Read the model definition and answer for the solid it produces. Units are mm, in the model's axes. Face numbers are marked on the shaded views. A direction names the side the tool comes from. Coordinates: 2 decimals unless noted, no trailing zeros. Loops run counter-clockwise (first coordinate to the right, second up) from the corner with the lowest first, then second, coordinate; pieces in that order, holes last.
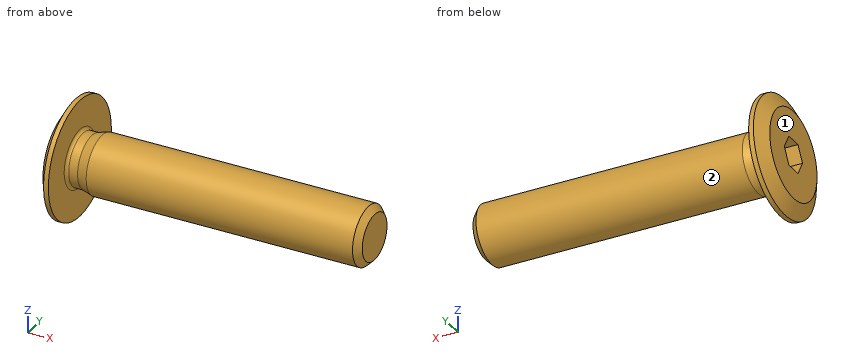
Autodesk Inventor part; units mm, degrees
ref_plane "YZ Plane" through (0, 0, 0) normal (1, 0, 0) x (0, 1, 0)
ref_plane "XZ Plane" through (0, 0, 0) normal (0, 1, 0) x (-1, 0, 0)
ref_plane "XY Plane" through (0, 0, 0) normal (0, 0, 1) x (1, 0, 0)
sketch "Sketch_1" plane through (0, 0, 0) normal (0, 0, 1) x (1, 0, 0)
  line L0 (20, 0) -> (-0.9, 0)
  line L1 (-0.9, 0) -> (-0.9, 3)
  line L2 (-0.9, 3) -> (-0.3226, 4)
  line L3 (-0.3226, 4) -> (0, 4)
  line L4 (0, 4) -> (0, 1.9852)
  arc A0 (0, 1.9852) -> (0.2, 1.7853) centre (0.2, 1.9853) ccw
  line L5 (0.2, 1.7853) -> (0.8, 1.7853)
  line L6 (0.8, 1.7853) -> (1.5, 2)
  line L7 (1.5, 2) -> (19.5705, 2)
  line L8 (19.5705, 2) -> (20, 1.5705)
  line L9 (20, 1.5705) -> (20, 0)
  line L10 (20, 0) -> (-0.9, 0)
revolve "Revolution1" add sketch "Sketch_1" angle 360 about axis through (20, 0, 0) along (1, 0, 0)
thread "Thread1"
sketch "Sketch2" plane through (-0.9, 0, 0) normal (-1, 0, 0) x (0, 0, 1)
  point P0 (0, 0)
hole "Hole1" at (-0.9, 0, 0) direction (1, 0, 0) diameter 2 depth 2.5 tip angle 120
sketch "Sketch_3" plane through (-0.9, 0, 0) normal (1, 0, 0) x (0, 0, -1)
  line L0 (-1, -0.5774) -> (0, -1.1547)
  line L1 (0, -1.1547) -> (1, -0.5774)
  line L2 (1, -0.5774) -> (1, 0.5774)
  line L3 (1, 0.5774) -> (0, 1.1547)
  line L4 (0, 1.1547) -> (-1, 0.5774)
  line L5 (-1, 0.5774) -> (-1, -0.5774)
extrude "Extrusion1" cut sketch "Sketch_3" along normal blind 2.5
properties part number "CBSTSR4-20"
Q1. Which of the six approach directions +Z, -Z, +X, -X, +Y, -Y give full straight-line access (tool end or side, diameter ignored) to the marked faces 1 and 2?
Findings below:
face 1: +Z, -Z, -X, +Y, -Y
face 2: +X
Q2. Flat-ended cylindrical pins translate along their axes: pin 1 Ø3 at (x, z) = (11.5, -2.5) entering from -Y; pin 2 Ø4 at (x, y) = (2.5, 2.5) entering from -Z; pin 3 Ø4 at (y, z) = (2, -1.5) entering from +X; pin 4 Ø3 at (x, z) = (15.5, 2) entering from +Y. Find the tip coordinate at first contact, or state that the pin passes through.
Findings below:
pin 1: stops at y = -1.73
pin 2: stops at z = -1.94
pin 3: stops at x = 20
pin 4: stops at y = 1.94
Q3. A cutting plane is placed at A-A (x = 1). Give the vertices of the cut face in (y, z).
Findings below:
outline: circle Ø3.69 at (0, 0); hole (-1.15, 0) - (-0.58, -1) - (0.58, -1) - (1.15, 0) - (0.58, 1) - (-0.58, 1) - close
Q4. Straight lines are drawn through the part: probe 1 along X at (y, z) = (-2.75, 0.5); probe 2 along Z at (x, y) = (1, 0.25); probe 3 along Z at (x, y) = (15.75, 0.25). For each, find the intervals that lie inside material, in ascending order.
Findings below:
probe 1: x = -0.9 to 0
probe 2: z = -1.83 to -1, 1 to 1.83
probe 3: z = -1.98 to 1.98
Q5. A cutting plane is placed at B-B (x = 12.25). Give the vertices of the cut face in (y, z).
Findings below:
outline: circle Ø4 at (0, 0)
